```python
from build123d import *

# Parameters (mm, degrees)
BOSS_EXTRUDE1_DEPTH     = 4.445
CUT_EXTRUDE1_REACH      = 13.535
CUT_EXTRUDE1_END_RADIUS = 41.91
SKETCH2_W               = 9.8425
SKETCH2_H               = 8.255
CUT_EXTRUDE3_REACH      = 14.779
CUT_EXTRUDE3_END_RADIUS = 43.18
SKETCH3_W               = 9.525
SKETCH3_H               = 8.255
CUT_EXTRUDE5_DEPTH      = 12.535347849
CUT_EXTRUDE5_DEPTH_BACK = 12.535347849


with BuildPart() as part:
    # Sketch1 → Boss-Extrude1 (new, symmetric)
    with BuildSketch(Plane.XY):
        with BuildLine():
            Line((-10.16, 0), (-10.16, 3.175))
            ThreePointArc((-10.16, 3.175), (0.312688289, 1.885753156), (10.16, -1.905))
            Line((10.16, -1.905), (10.16, -3.175))
            Line((10.16, -3.175), (0, -3.175))
            Line((0, -3.175), (0, 0))
            Line((0, 0), (-10.16, 0))
        make_face()
    extrude(amount=BOSS_EXTRUDE1_DEPTH, both=True)

    # Cut-Extrude1: up to this cylinder (the profile starts inside it)
    cut_extrude1_end = Plane(origin=(-10.16, -40.005, 0), z_dir=(0, 0, -1)) * Cylinder(CUT_EXTRUDE1_END_RADIUS, 111.89, mode=Mode.PRIVATE)
    # Sketch2 → Cut-Extrude1 (cut, up to the surface)
    with BuildSketch(Plane.XZ, mode=Mode.PRIVATE) as cut_extrude1_sk1:
        with Locations((-4.92125, 0)):
            Rectangle(SKETCH2_W, SKETCH2_H)
    cut_extrude1_tool1 = extrude(cut_extrude1_sk1.sketch, amount=-CUT_EXTRUDE1_REACH, mode=Mode.PRIVATE) & cut_extrude1_end
    add(cut_extrude1_tool1.solids().sort_by_distance((-4.92125, 0, 0))[0], mode=Mode.SUBTRACT)

    # Cut-Extrude3: up to this cylinder (the profile starts inside it)
    cut_extrude3_end = Plane(origin=(-10.16, -41.275, 0), z_dir=(0, 0, -1)) * Cylinder(CUT_EXTRUDE3_END_RADIUS, 116.918, mode=Mode.PRIVATE)
    # Sketch3 → Cut-Extrude3 (cut, up to the surface)
    with BuildSketch(Plane.XZ.offset(3.175), mode=Mode.PRIVATE) as cut_extrude3_sk1:
        with Locations((5.08, 0)):
            Rectangle(SKETCH3_W, SKETCH3_H)
    cut_extrude3_tool1 = extrude(cut_extrude3_sk1.sketch, amount=-CUT_EXTRUDE3_REACH, mode=Mode.PRIVATE) & cut_extrude3_end
    add(cut_extrude3_tool1.solids().sort_by_distance((5.08, -3.175, 0))[0], mode=Mode.SUBTRACT)

    # Sketch7 → Cut-Extrude5 (cut, two sides)
    with BuildSketch(Plane(origin=(0, 0, 0), x_dir=(1, 0, 0), z_dir=(0, 1, 0))) as cut_extrude5_sk:
        Polygon((10.16, 3.175), (0, -4.445), (10.16, -4.445), align=None)
    extrude(amount=CUT_EXTRUDE5_DEPTH, mode=Mode.SUBTRACT)
    extrude(cut_extrude5_sk.sketch, amount=-CUT_EXTRUDE5_DEPTH_BACK, mode=Mode.SUBTRACT)


solid = part.part
```
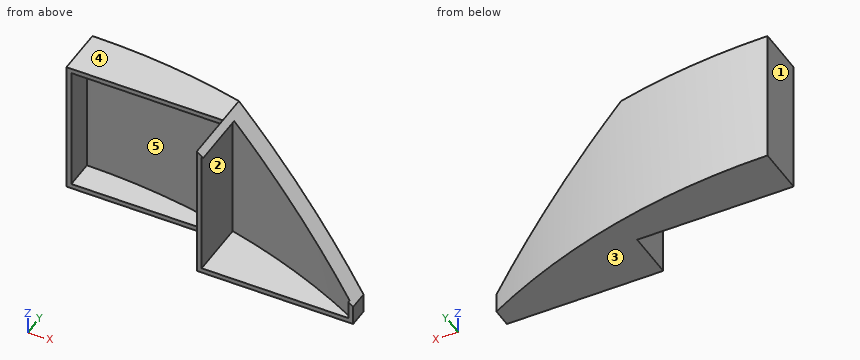
The model under review builds one solid part; all positions refer to its coordinate system, in mm. Face numbers are marked on the shaded views. A direction names the side the tool comes from. Round coordinates to 2 decimals unless told otherwise and drop trailing zeros. Order: outer loops, then holes, each group sorted by start corner. A loop starts at its lowest first (then second) coordinate and runs counter-clockwise, first axis right, second up.
Item 1: To check wall thickness, follow probe 1 along X at (y, z) = (-1.5, -3.5); probe 2 along Z at (x, y) = (-0.25, 0.5) (1 decimal); probe 3 along X at (y, z) = (-1, 3.5). State the ranges of each line that lie inside material, in increasing order.
Working result:
probe 1: x = 0 to 0.32, 6.65 to 9.38
probe 2: z = -4.4 to -4.1, 4.1 to 4.4
probe 3: x = 0 to 0.32
Item 2: Add section A-A, the plane y = 1.5. State the section outline as (x, z) points (1 decimal).
Working result:
outline: (-10.2, -4.4) - (1.7, -4.4) - (1.7, 3.1) - (0, 4.4) - (-10.2, 4.4) - close; hole (-9.8, -4.1) - (-4.3, -4.1) - (-4.3, 4.1) - (-9.8, 4.1) - close
Item 3: Machinability: for the marked faces 4 and 5, which of the approach directions +Z, -Z, +X, -X, +Y, -Y give a long, thin tool a straight path to every point of the face, cutting with its end or side? Answer none if there is none.
Working result:
face 4: +Z, +X, -X, +Y, -Y
face 5: -Y
Item 4: For pin 1 (3 mm diameter, centred on x = -5.5, z = -0.5, fed in from -Y); pin 2 (1.5 mm diameter, centred on x = -3, z = -1.5, fed in from -Y); pin 3 (2 mm diameter, centred on y = -2.5, z = 0.5, fed in from +X), all flat-tipped, find the tip position at first contact; note any pin that passes through.
Working result:
pin 1: stops at y = 1.45
pin 2: stops at y = 1.15
pin 3: stops at x = 0.32
Item 5: Draft analysis for pull direction Z (two halves, no side actions). For the marked faces 1, 2 and 3, state which applies: released by +Z, released by -Z, zero draft, split by the parting line, or undercut.
Working result:
face 1: zero draft
face 2: undercut
face 3: released by -Z
